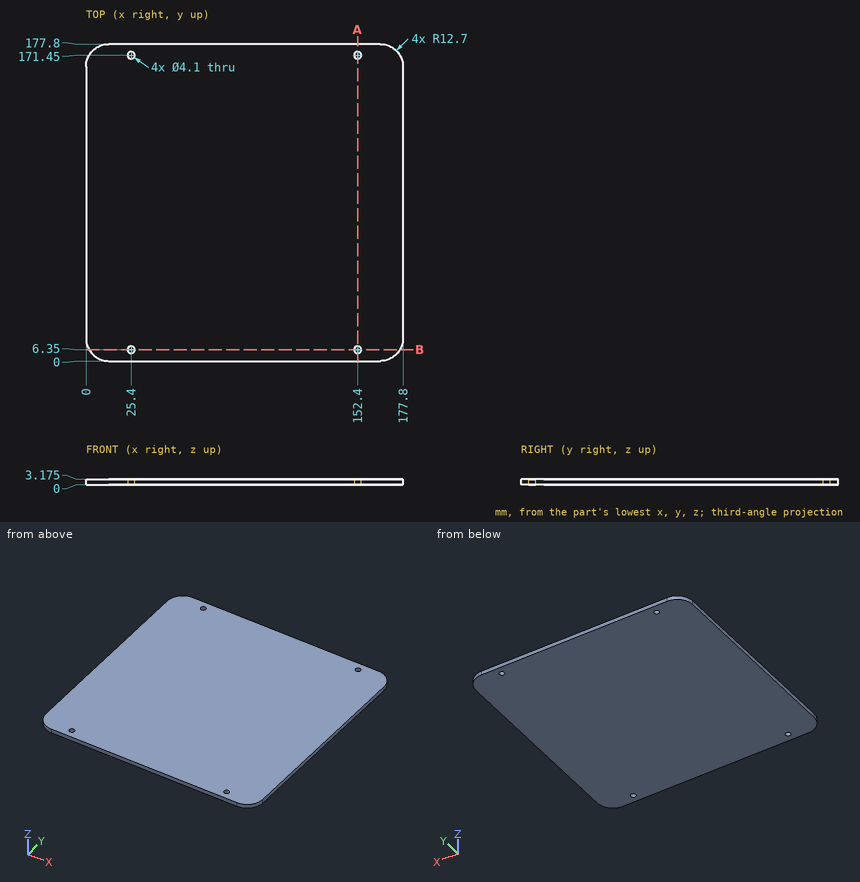
Design review of the part shown in the three views and the two pictorial views. Dimensions are in mm from the part's minimum x, y and z. Give positions to 0.01 mm unless a question says otherwise; leave off trailing zeros. Loops run counter-clockwise (first coordinate to the right, second up) from the corner with the lowest first, then second, coordinate; pieces in that order, holes last. Notation, with made-up numbers: M -6.5,-38.75 L 40.5,-38.75 A23 cw 40.5,-25.75 Z; hole C 47.5,-17 d7. An arc over 180 degrees is marked long. Put each result on its own line as item: value. Start each with the question number.
(1) Wall thickness on L1, parallel to Y at x = 152.4, z = 1.1; L2, parallel to Y at x = 27, z = 2.2; L3, parallel to X at y = 6.35, z = 1.25: over which ranges is each line inside the solid? List them lowest first.
(2) For pin 1 (3.5 mm diameter, centred on x = 25.4, y = 6.35, fed in from +Z), flat-tipped, find the tip position at first contact; note if it passes through.
(3) Add section A-A, the plane x = 152.4. Write out the cut boundary in (y, z) (3 decimals), then the cut area to 3 significant figures.
(4) Add section B-B, the plane y = 6.35. Write out the cut boundary in (x, z) (3 decimals).
Result:
1. L1: y = 0 to 4.3, 8.4 to 169.4, 173.5 to 177.8
1. L2: y = 0 to 5.07, 7.63 to 170.17, 172.73 to 177.8
1. L3: x = 1.7 to 23.35, 27.45 to 150.35, 154.45 to 176.1
2. pin 1: passes through
3. outline: M 0,0 L 4.3,0 L 4.3,3.175 L 0,3.175 Z; M 8.4,0 L 169.4,0 L 169.4,3.175 L 8.4,3.175 Z; M 173.5,0 L 177.8,0 L 177.8,3.175 L 173.5,3.175 Z
3. area: 538 mm^2
4. outline: M 1.701,0 L 23.35,0 L 23.35,3.175 L 1.701,3.175 Z; M 27.45,0 L 150.35,0 L 150.35,3.175 L 27.45,3.175 Z; M 154.45,0 L 176.099,0 L 176.099,3.175 L 154.45,3.175 Z
